The model under review builds one solid part; all positions refer to its coordinate system, in mm. Face numbers are marked on the shaded views. Round coordinates to 2 decimals unless told otherwise and drop trailing zeros. Write each loop counter-clockwise with the first axis right and the second up, starting at its lowest first coordinate (ties: lowest second). Pieces come first, ordered by that corner, then holes. Notation, with made-up numbers: (-2.5, 77) -> (33.5, 77) arc R26 cw to (33.5, 94) -> close; hole circle Ø7 at (-25.5, 43). An arc over 180 degrees is marked (long way). Return JSON: item names as keys, results as strings. Group by question number.
1. Mouldability with a two-part tool opening along Y and no side actions: class the marked faces 1, 2, 3 and 4 as pulls with the +Y half, pulls with the -Y half, needs draft (parallel to the pull), parting line crosses it, or undercut.
2. For line 1 along Y through (x, z) = (41, 2); line 2 along X through (y, z) = (24, 5); line 3 along Y through (x, z) = (38.5, 4.5), list the stretches that pass through material, from the lowest coordinate up. Write a range as from..to.
3. Take a section at A-A, the plane x = 41. Write out the cut boundary in (y, z).
from build123d import *

# Parameters (mm, degrees)
F0_W     = 40
F0_H     = 8
F1_DEPTH = 56
F2_R     = 3
F3_DEPTH = 11.1


with BuildPart() as f1:
    # F0 (on Right) → F1 (new body)
    with BuildSketch(Plane.YZ):
        with Locations((21.365855, 4)):
            Rectangle(F0_W, F0_H)
    extrude(amount=F1_DEPTH)

    # F2 (on face) → F3 (cut)
    with BuildSketch(Plane(origin=(0, 0, 0), x_dir=(1, 0, 0), z_dir=(0, 0, -1))):
        with Locations((41, -23.152475)):
            Circle(F2_R)
    extrude(amount=-F3_DEPTH, mode=Mode.SUBTRACT)


solid = f1.part
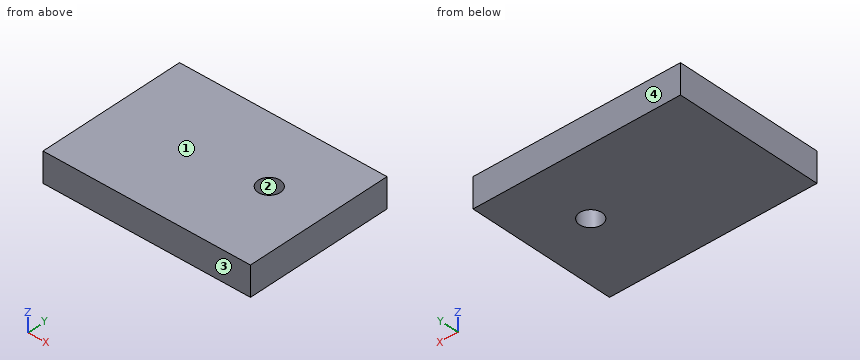
Output:
{
 "1": {"face 1": "needs draft", "face 2": "undercut", "face 3": "pulls with the -Y half", "face 4": "pulls with the +Y half"},
 "2": {"line 1": "y = 1.37..20.15, 26.15..41.37", "line 2": "x = 0..38.12, 43.88..56", "line 3": "y = 1.37..21.49, 24.81..41.37"},
 "3": {"outline": "(1.37, 0) -> (20.15, 0) -> (20.15, 8) -> (1.37, 8) -> close; (26.15, 0) -> (41.37, 0) -> (41.37, 8) -> (26.15, 8) -> close"}
}
